Here's how the part is built. I have some questions about the finished solid (model axes, mm). A direction names the side the tool comes from. Coordinates: 2 decimals unless noted, no trailing zeros. Loops run counter-clockwise (first coordinate to the right, second up) from the corner with the lowest first, then second, coordinate; pieces in that order, holes last. Notation, with made-up numbers: M 29.25,40.5 L 49.25,40.5 A17 cw 49.25,47.5 Z; hole C -37.75,6 d10. An arc over 180 degrees is marked long. Use CSV: the item, a comma, the result in double quotes. Start each with the question number.
Q1. Which directions (+Z, -Z, +X, -X, +Y, -Y) give clear straight access to the entire face, cutting with the end or side of a thin tool? Please do faces 4 (the flat face through (-9.525, -42, 3)), 5 (the flat face through (-11, 0, 0)), 6 (the flat face through (9.525, -42, 3)), 7 (the flat face through (25, 26, 6.35)), 8 (the flat face through (-42, 9.525, 3)).
Q2. If we mould it in two halves opening along X, with no side actions, what happens to faces 1 (the flat face through (-9.525, 41, 3)), 2 (the flat face through (73.025, 0, 3)), 3 (the cylindrical face through (-7.956, 7.296, 15.653))? For each: +X half, -X half, draft (parallel to the pull), parting line (faces both ways), or undercut.
Q3. Please list where these lines run through material, in increasing order: probe 1 along Y at (x, z) = (-51, 3.5) (3 decimals); probe 2 along Y at (x, z) = (0, 14.5) (3 decimals); probe 3 along Y at (x, z) = (6.5, 26). Write a range as [from, to].
Q4. If we section it at A-A (x = -52.5): Please give me the cut outline in (y, z) (3 decimals), and give its area (3 significant figures).
Q5. For pin 1 Ø20 at (x, y) = (-26, -23) entering from -Z; pin 2 Ø1.5 at (x, z) = (-4, 15) entering from -Y; pin 3 Ø21 at (x, y) = (-3, 65.5) entering from +Z; pin 4 Ø1.5 at (x, y) = (-2.5, -12) entering from -Z, each with a flat end and sliding along its axis, tell me the tip position at first contact or that it passes through.
from build123d import *

# Parameters (mm, degrees)
F0_W     = 19.05
F0_H     = 63.5
F0_W_2   = 63.5
F0_H_2   = 19.05
F1_DEPTH = 6.35
F2_R     = 10.795
F3_DEPTH = 25.4
F4_DEPTH = 6.35


# Not quite as in the source:
# - a fillet or chamfer that OpenCascade refuses, or shapes differently, is made with other operations: its cross-section is extruded or revolved along the edge and cut away or added


with BuildPart() as f1:
    # F0 (on Top) → F1 (new body)
    with BuildSketch(Plane.XY):
        with Locations((0, 41.275)):
            Rectangle(F0_W, F0_H)
        with Locations((-41.275, 0)):
            Rectangle(F0_W_2, F0_H_2)
        Rectangle(F0_W, F0_H_2)
        with Locations((41.275, 0)):
            Rectangle(F0_W_2, F0_H_2)
        with Locations((0, -41.275)):
            Rectangle(F0_W, F0_H)
    extrude(amount=F1_DEPTH)

    # F2 (on face) → F3 (join)
    with BuildSketch(Plane.XY.offset(6.35)):
        with BuildLine():
            ThreePointArc((49.8990418245, -9.525), (50.5742588907, -4.7837576923), (50.8, 0))
            ThreePointArc((50.8, 0), (50.5742588907, 4.7837576923), (49.8990418245, 9.525))
            Line((49.8990418245, 9.525), (9.525, 9.525))
            Line((9.525, 9.525), (9.525, 49.8990418245))
            ThreePointArc((9.525, 49.8990418245), (0, 50.8), (-9.525, 49.8990418245))
            Line((-9.525, 49.8990418245), (-9.525, 9.525))
            Line((-9.525, 9.525), (-49.8990418245, 9.525))
            ThreePointArc((-49.8990418245, 9.525), (-50.8, 0), (-49.8990418245, -9.525))
            Line((-49.8990418245, -9.525), (-9.525, -9.525))
            Line((-9.525, -9.525), (-9.525, -49.8990418245))
            ThreePointArc((-9.525, -49.8990418245), (0, -50.8), (9.525, -49.8990418245))
            Line((9.525, -49.8990418245), (9.525, -9.525))
            Line((9.525, -9.525), (49.8990418245, -9.525))
        make_face()
        Circle(F2_R, mode=Mode.SUBTRACT)
        with BuildLine():
            ThreePointArc((-49.8990418245, -9.525), (-35.9210244843, -35.9210244843), (-9.525, -49.8990418245))
            Line((-9.525, -49.8990418245), (-9.525, -9.525))
            Line((-9.525, -9.525), (-49.8990418245, -9.525))
        make_face()
        with BuildLine():
            Line((-9.525, 9.525), (-9.525, 49.8990418245))
            ThreePointArc((-9.525, 49.8990418245), (-35.9210244843, 35.9210244843), (-49.8990418245, 9.525))
            Line((-49.8990418245, 9.525), (-9.525, 9.525))
        make_face()
        with BuildLine():
            Line((9.525, 9.525), (49.8990418245, 9.525))
            ThreePointArc((49.8990418245, 9.525), (35.9210244843, 35.9210244843), (9.525, 49.8990418245))
            Line((9.525, 49.8990418245), (9.525, 9.525))
        make_face()
        with BuildLine():
            ThreePointArc((9.525, -49.8990418245), (35.9210244843, -35.9210244843), (49.8990418245, -9.525))
            Line((49.8990418245, -9.525), (9.525, -9.525))
            Line((9.525, -9.525), (9.525, -49.8990418245))
        make_face()
    extrude(amount=F3_DEPTH)

    # F4 (cut, through all): a face of the model
    f4_faces = [f1.faces().sort_by_distance(p)[0] for p in [
        (0, 0, 6.35),
    ]]
    extrude(f4_faces, amount=-F4_DEPTH, mode=Mode.SUBTRACT)

    # F5: fillet of radius 38.1 on 1 edges, made by hand

    # F5_s1 → F5_t2 (revolve, cut)
    with BuildSketch(Plane(origin=(0, 0, 0), x_dir=(0, 0, 1), z_dir=(-0.9822646028, -0.1875, 0))):
        with BuildLine():
            ThreePointArc((6.35, -50.8), (24.7585197333, -36.8760207718), (31.75, -14.8789755157))
            Line((31.75, -14.8789755157), (32.512, -14.8789755157))
            Line((32.512, -14.8789755157), (32.512, -50.8))
            Line((32.512, -50.8), (31.75, -51.562))
            ThreePointArc((31.75, -51.562), (19.05, -51.562), (6.604, -51.5184204897))
            Line((6.604, -51.5184204897), (6.35, -50.8))
        make_face()
    revolve(axis=Axis((0, 0, 31.75), (0, 0, 1)), mode=Mode.SUBTRACT)


solid = f1.part
Results below:
1,face 4,"-Z, -X, -Y"
1,face 5,"-Z, +X, -X, +Y, -Y"
1,face 6,"-Z, +X, -Y"
1,face 7,"-Z, +X, +Y"
1,face 8,"-Z, -X, +Y"
2,face 1,"-X half"
2,face 2,"+X half"
2,face 3,"undercut"
3,probe 1,"[-9.525, 9.525]"
3,probe 2,"[-46.768, -10.795], [10.795, 46.768]"
3,probe 3,"[-34.4, -8.62], [8.62, 34.4]"
4,outline,"M -9.525,0 L 9.525,0 L 9.525,6.35 L -9.525,6.35 Z"
4,area,"121 mm^2"
5,pin 1,"z = 6.35"
5,pin 2,"y = -46.76"
5,pin 3,"z = 6.35"
5,pin 4,"z = 0"
